Answer from the drawing. Dimensions are ordinates in mm from the lowest x, y and z of the part. A direction names the side the tool comes from. Coordinates: 2 decimals unless noted, no trailing zeros. Order: outer loops, then holes, each group sorted by start corner. A loop starts at its lowest first (then second) coordinate and runs counter-clockwise, first axis right, second up. Notation, with made-up numbers: M 48.5,25 L 106.5,25 A20 ccw 106.5,33 Z; hole C 47.25,-14 d6. An arc over 180 degrees is marked long. One line per question, with ' | ' between items. Start each with the question number.
1) The mould has two halves that part along Y. Classify the marked faces 1, 2 and 3: +Y half, -Y half, draft (parallel to the pull), parting line (faces both ways), or undercut.
2) Find section C-C, the plane y = 12.5. Write down the section's boundary in (x, z), plus the area to 3 significant figures.
3) Find section A-A, the plane z = 45. Count the separate pieces of the cut face and the enclosed holes in it, plus the area to 3 significant figures.
4) Given P1, Ø10, axis at x = 15, y = 30, coming from the -Z side; P2, Ø1.5, axis at x = 28, z = 23, coming from the +Y side; P3, Ø4, axis at x = 30.5, z = 45.5, coming from the -Y side; P4, Ø18, axis at y = 45, z = 45, coming from the -X side, each flat-ended and moving along its own axis, determine where each tip first touches the part or whether it passes through.
5) A tool of negligible diameter and unlimited length cuts with its end or side. For the marked faces 4, 5 and 6, from which of +Z, -Z, +X, -X, +Y, -Y can it reach the whole face along a straight path? Write none if from no direction.
6) Consider probe 1 along Y at (x, z) = (84.5, 45); probe 2 along Z at (x, y) = (14.5, 45); probe 3 along Y at (x, z) = (43, 45). Determine where each line is inside the solid, lowest interval first.
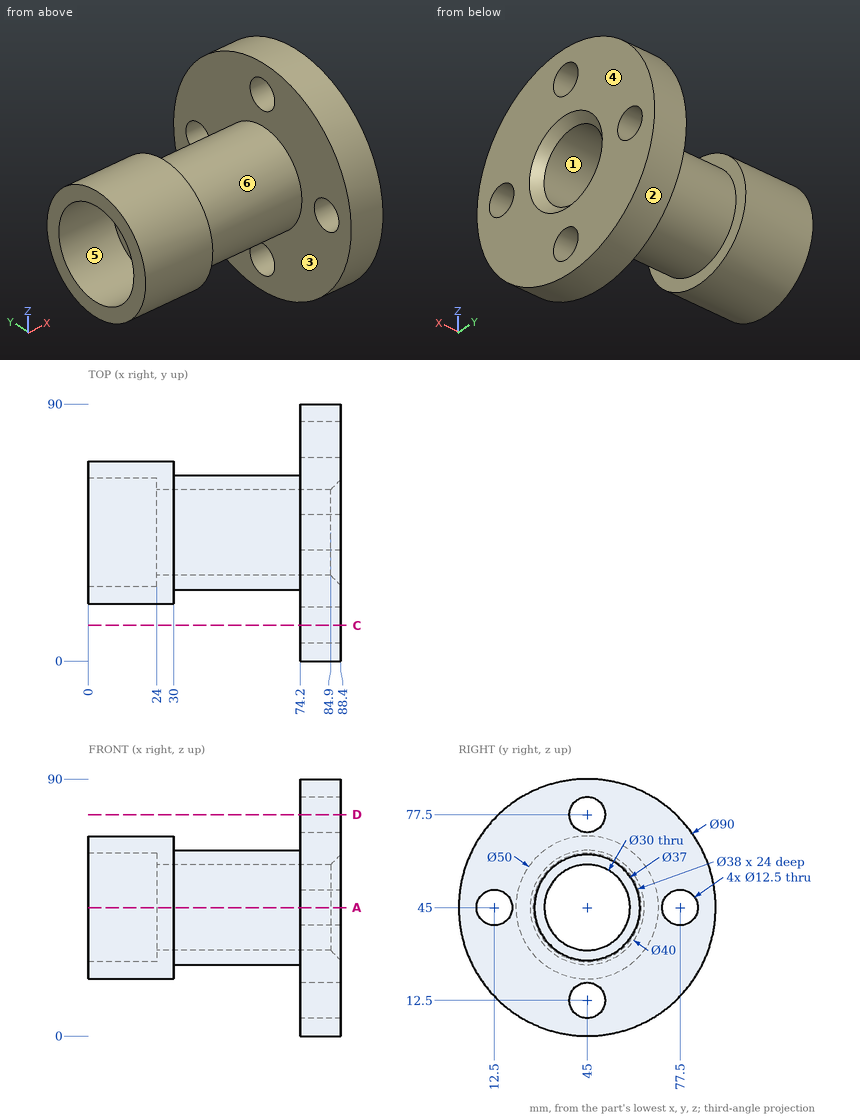
Report:
1) face 1: undercut | face 2: parting line | face 3: draft
2) outline: M 74.2,13.88 L 88.4,13.88 L 88.4,38.75 L 74.2,38.75 Z; M 74.2,51.25 L 88.4,51.25 L 88.4,76.12 L 74.2,76.12 Z | area: 706 mm^2
3) separate pieces: 4 | enclosed holes: 0 | area: 1,330 mm^2
4) P1: stops at z = 22.09 | P2: stops at y = 58.17 | P3: stops at y = 20 | P4: passes through
5) face 4: +Z, -Z, +X, +Y, -Y | face 5: -X | face 6: none
6) probe 1: y = 0 to 6.25, 18.75 to 30, 60 to 71.25, 83.75 to 90 | probe 2: z = 20 to 26, 64 to 70 | probe 3: y = 25 to 30, 60 to 65
